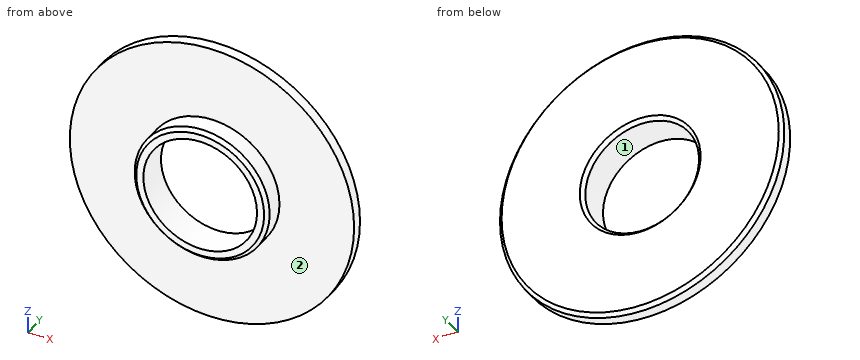
```python
from build123d import *

# Parameters (mm, degrees)
SMUSSO1_SIZE = 0.5


with BuildPart() as part:
    # Schizzo1 → Rivoluzione1 (revolve)
    with BuildSketch(Plane.XY):
        Polygon((8, 0), (20, 0), (20, -2), (9.5, -2), (9.5, -5), (8, -5), align=None)
    revolve(axis=Axis((0, -42.973726115, 0), (0, 1, 0)))

    # Smusso1
    smusso1_edges = [part.edges().sort_by_distance(p)[0] for p in [
        (-9.5, -5, 0),
        (-20, 0, 0),
        (-8, 0, 0),
    ]]
    chamfer(smusso1_edges, length=SMUSSO1_SIZE)


solid = part.part
```
Here's how the part is built. I have some questions about the finished solid (model axes, mm). Face numbers are marked on the shaded views. Give positions to 0.01 mm unless a question says otherwise; leave off trailing zeros. Loops run counter-clockwise (first coordinate to the right, second up) from the corner with the lowest first, then second, coordinate; pieces in that order, holes last. Notation, with made-up numbers: (83.5, 55) -> (136.5, 55) arc R27 cw to (136.5, 71) -> close; hole circle Ø9 at (77, -27). An arc over 180 degrees is marked (long way). Use one line per item in the form item = value. Start each with the question number.
1) Thinking about a two-plate mould opening in Z: for the marked faces 1 and 2, which applies, +Z half, -Z half, draft (parallel to the pull), parting line (faces both ways), or undercut?
2) Imagine slicing it at B-B (z = 0). Please give me the cut outline in (x, y).
3) Please list where these lines run through material, in increasing order: line 1 along X through (y, z) = (-2.8, 0); line 2 along X through (y, z) = (-1.65, 0).
4) For P1, Ø2, axis at x = 12.5, z = -3, coming from the -Y side; P2, Ø3, axis at x = -7.5, y = -3, coming from the +Z side; P3, Ø3, axis at x = -4, z = 3.5, coming from the -Y side, each with a flat end and sliding along its axis, tell me the tip position at first contact or that it passes through.
5) Imagine slicing it at A-A (x = 0). Please give me the cut outline in (y, z).
6) Imagine slicing it at C-C (y = -2.9). Please give me the cut outline in (x, z), then the cut area to 3 significant figures.
Check values:
q1.face_1 = undercut
q1.face_2 = draft
q2.outline = (-20, -2) -> (-9.5, -2) -> (-9.5, -4.5) -> (-9, -5) -> (-8, -5) -> (-8, -0.5) -> (-8.5, 0) -> (-19.5, 0) -> (-20, -0.5) -> close; (8, -5) -> (9, -5) -> (9.5, -4.5) -> (9.5, -2) -> (20, -2) -> (20, -0.5) -> (19.5, 0) -> (8.5, 0) -> (8, -0.5) -> close
q3.line_1 = -9.5 to -8, 8 to 9.5
q3.line_2 = -20 to -8, 8 to 20
q4.P1 = -2
q4.P2 = 18.95
q4.P3 = through
q5.outline = (-5, -9) -> (-4.5, -9.5) -> (-2, -9.5) -> (-2, -20) -> (-0.5, -20) -> (0, -19.5) -> (0, -8.5) -> (-0.5, -8) -> (-5, -8) -> close; (-5, 8) -> (-0.5, 8) -> (0, 8.5) -> (0, 19.5) -> (-0.5, 20) -> (-2, 20) -> (-2, 9.5) -> (-4.5, 9.5) -> (-5, 9) -> close
q6.outline = circle Ø19 at (0, 0); hole circle Ø16 at (0, 0)
q6.area = 82.5 mm^2
